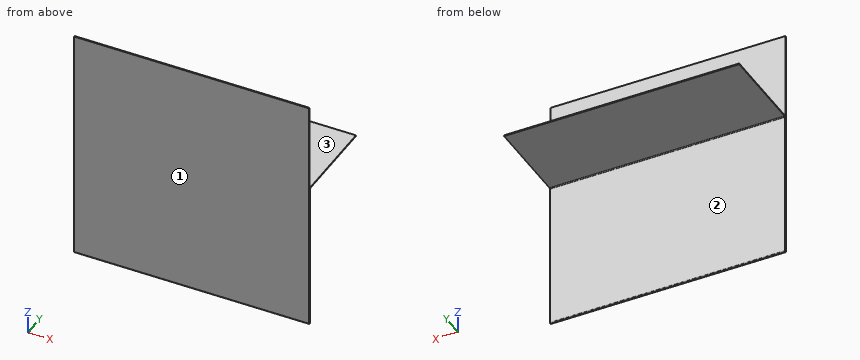
from build123d import *

# Parameters (mm, degrees)
SKETCH1_W                    = 198
SKETCH1_H                    = 125
BASE_FLANGE1_DEPTH           = 0.7366
EDGE_FLANGE1_STRIP_W         = 4.4196
EDGE_FLANGE1_STRIP_H         = 0.7366
EDGE_FLANGE1_STRIP_CUT_DEPTH = 198
EDGE_FLANGE1_DEPTH           = 198
HEM1_START                   = -99
HEM1_DEPTH                   = 198
HEM1_2_DEPTH                 = 198


with BuildPart() as part:
    # Base-Flange1: sheet metal written as solids
    # Sketch1 → Base-Flange1 (new body)
    with BuildSketch(Plane(origin=(0, 0, 0), x_dir=(1, 0, 0), z_dir=(0, 1, 0))):
        with Locations((0, 32.491501416)):
            Rectangle(SKETCH1_W, SKETCH1_H)
    extrude(amount=-BASE_FLANGE1_DEPTH)

    # Edge-Flange1: sheet metal written as solids
    # Edge-Flange1 strip (on a plane across the edge) → Edge-Flange1 strip cut (cut)
    with BuildSketch(Plane(origin=(-99, 0, 30.008498584), x_dir=(0, 0, -1), z_dir=(1, 0, 0))):
        with Locations((-1.4732, -0.3683)):
            Rectangle(EDGE_FLANGE1_STRIP_W, EDGE_FLANGE1_STRIP_H)
    extrude(amount=EDGE_FLANGE1_STRIP_CUT_DEPTH, mode=Mode.SUBTRACT)

    # Edge-Flange1 section (on a plane across the edge) → Edge-Flange1 (add)
    with BuildSketch(Plane(origin=(-99, 0, 30.008498584), x_dir=(0, 0, -1), z_dir=(1, 0, 0))):
        with BuildLine():
            Line((-0.7366, 0.7366), (-0.7366, 74.4732))
            Line((-0.7366, 74.4732), (0, 74.4732))
            Line((0, 74.4732), (0, 0.7366))
            ThreePointArc((0, 0.7366), (0.215745145, 0.215745145), (0.7366, 0))
            Line((0.7366, 0), (0.7366, -0.7366))
            ThreePointArc((0.7366, -0.7366), (-0.30510971, -0.30510971), (-0.7366, 0.7366))
        make_face()
    extrude(amount=EDGE_FLANGE1_DEPTH)

    # Hem1: read off the stored shape, not the designer's step
    # Hem1 outline → Hem1 (cut)
    with BuildSketch(Plane.YZ.offset(HEM1_START)):
        with BuildLine():
            ThreePointArc((0, -94.204901416), (-0.212984467, -94.743143722), (-0.7366, -94.98991069))
            Line((-0.7366, -94.98991069), (-0.7366, -94.991501416))
            Line((-0.7366, -94.991501416), (0, -94.991501416))
            Line((0, -94.991501416), (0, -94.204901416))
        make_face()
    extrude(amount=HEM1_DEPTH, mode=Mode.SUBTRACT)

    # Hem1 2 outline → Hem1 2 (add)
    with BuildSketch(Plane.YZ.offset(HEM1_START)):
        with BuildLine():
            Line((-0.8366, 105.008498584), (-1.5732, 105.008498584))
            Line((-1.5732, 105.008498584), (-1.5732, -94.204901416))
            ThreePointArc((-1.5732, -94.204901416), (-1.324842306, -94.778516949), (-0.7366, -94.98991069))
            Line((-0.7366, -94.98991069), (-0.7366, -94.204901416))
            ThreePointArc((-0.7366, -94.204901416), (-0.7866, -94.254901416), (-0.8366, -94.204901416))
            Line((-0.8366, -94.204901416), (-0.8366, 105.008498584))
        make_face()
    extrude(amount=HEM1_2_DEPTH)


solid = part.part
The model under review builds one solid part; all positions refer to its coordinate system, in mm. Face numbers are marked on the shaded views. A direction names the side the tool comes from. Round coordinates to 2 decimals unless told otherwise and drop trailing zeros. Loops run counter-clockwise (first coordinate to the right, second up) from the corner with the lowest first, then second, coordinate; pieces in that order, holes last. Notation, with made-up numbers: (89.5, -7.5) -> (148.5, -7.5) arc R19 cw to (148.5, 16.5) -> close; hole circle Ø8 at (73.25, 18). An arc over 180 degrees is marked (long way). Answer as CSV lines item,"result".
1) Add section A-A on z = 21. Write out the cut boundary in (x, y).
Geometry results:
outline,"(-99, -1.57) -> (99, -1.57) -> (99, -0.84) -> (-99, -0.84) -> close; (-99, -0.74) -> (99, -0.74) -> (99, 0) -> (-99, 0) -> close"
2) To check wall thickness, follow line 1 along Y through (x, z) = (61, 39.5); line 2 along Z through (x, y) = (19, 29.5). State the ranges of each line that lie inside material, in increasing order. Write a range as from..to.
Geometry results:
line 1,"y = -1.57..-0.84"
line 2,"z = 30.01..30.75"
3) Add section C-C on y = 54.5. Write out the cut boundary in (x, z).
Geometry results:
outline,"(-99, 30.01) -> (99, 30.01) -> (99, 30.75) -> (-99, 30.75) -> close"
4) Add section D-D on z = 42. Write out the cut boundary in (x, y), plus the area to 3 significant figures.
Geometry results:
outline,"(-99, -1.57) -> (99, -1.57) -> (99, -0.84) -> (-99, -0.84) -> close"
area,"146 mm²"
5) For P1, Ø5, axis at x = -65, z = 7, coming from the +Y side; P2, Ø2, axis at x = 9.5, y = 36, coming from the -Z side; P3, Ø6, axis at x = 40, y = 55, coming from the +Z side, all flat-tipped, find the tip position at first contact; note any pin that passes through.
Geometry results:
P1,"stops at y = 0"
P2,"stops at z = 30.01"
P3,"stops at z = 30.75"
6) Add section B-B on x = 65. Write out the cut boundary in (y, z), plus the area to 3 significant figures.
Geometry results:
outline,"(-1.57, -94.2) arc R0.79 ccw to (0, -94.2) -> (0, 29.27) arc R0.74 cw to (0.74, 30.01) -> (74.47, 30.01) -> (74.47, 30.75) -> (0.74, 30.75) arc R1.47 ccw to (-0.74, 29.27) -> (-0.74, -94.2) arc R0.05 cw to (-0.84, -94.2) -> (-0.84, 105.01) -> (-1.57, 105.01) -> close"
area,"294 mm²"
7) Tool access review of the marked faces 1, 2 and 3: name each direction out of +Z, -Z, +X, -X, +Y, -Y from which nothing blocks a thin tool from reaching the whole face with its end or side.
Geometry results:
face 1,"+Z, -Z, +X, -X, -Y"
face 2,"-Z, +X, -X, +Y"
face 3,"+Z, +X, -X, +Y"
